Here's how the part is built. I have some questions about the finished solid (model axes, mm). A direction names the side the tool comes from. Give positions to 0.01 mm unless a question says otherwise; leave off trailing zeros. Order: outer loops, then holes, each group sorted by start corner. A loop starts at its lowest first (then second) coordinate and runs counter-clockwise, first axis right, second up. Notation, with made-up numbers: (88.25, 1) - (104.25, 1) arc R17 cw to (104.25, 15) - close; hole circle Ø3 at (88, 36.5). An arc over 180 degrees is marked (long way). One line per question, with ' | ' between items.
Autodesk Inventor part; units mm, degrees
ref_plane "YZ Plane" through (0, 0, 0) normal (1, 0, 0) x (0, 1, 0)
ref_plane "XZ Plane" through (0, 0, 0) normal (0, 1, 0) x (-1, 0, 0)
ref_plane "XY Plane" through (0, 0, 0) normal (0, 0, 1) x (1, 0, 0)
sketch "Sketch1" plane through (0, 0, 0) normal (0, 1, 0) x (-1, 0, 0)
  line L0 (52, 58.6471) -> (-48, 58.6471)
  line L1 (-48, 58.6471) -> (-48, -16.3529)
  line L2 (-48, -16.3529) -> (52, -16.3529)
  line L3 (52, -16.3529) -> (52, 58.6471)
  point P0 (0, 0)
  dimension "d0" = 100
  dimension "d1" = 75
extrude "Extrusion1" add sketch "Sketch1" along normal blind 60
sketch "Sketch2" plane through (0, 60, 0) normal (0, 1, 0) x (1, 0, 0)
  line L0 (-47, -53.6471) -> (43, -53.6471)
  line L1 (43, -53.6471) -> (43, 11.3529)
  line L2 (43, 11.3529) -> (-47, 11.3529)
  line L3 (-47, 11.3529) -> (-47, -53.6471)
  line L4 (-52, 16.3529) -> (-52, -58.6471)
  line L5 (-52, -58.6471) -> (48, -58.6471)
  line L6 (48, 16.3529) -> (-52, 16.3529)
  line L7 (48, -58.6471) -> (48, 16.3529)
  point P0 (0, 0)
  dimension "d4" = 5
  dimension "d5" = 5
  dimension "d6" = 5
  dimension "d7" = 5
extrude "Extrusion2" cut sketch "Sketch2" against normal blind 59 contours L3 L2 L1 L0
sketch "Sketch3" plane through (48, 0, -16.3529) normal (0, 0, -1) x (-1, 0, 0)
  circle A0 centre (48, 60) radius 13
  point P0 (48, 0)
  dimension "d10" = 26
  dimension "d11" = 60
sketch "Sketch13" plane through (0, 1, 0) normal (0, 1, 0) x (1, 0, 0)
  line L0 (-47, -53.6471) -> (-47, 11.3529)
  line L1 (43, 11.3529) -> (43, -53.6471)
  line L2 (-47, 11.3529) -> (43, 11.3529)
  line L3 (43, 11.3529) -> (43, -13.6471)
  line L4 (43, -13.6471) -> (-47, -13.6471)
  line L5 (-47, -13.6471) -> (-47, 11.3529)
  point P0 (0, 0)
  dimension "d44" = 25
extrude "Extrusion14" add sketch "Sketch13" along normal blind 59
sketch "Sketch14" plane through (-47, 1, 13.6471) normal (0, 0, 1) x (1, 0, 0)
  line L0 (0, 59) -> (90, 59)
  circle A0 centre (47, 59) radius 23.505
  point P0 (47, -1)
  dimension "d47" = 47.01
extrude "Extrusion15" cut sketch "Sketch14" against normal blind 12.1
sketch "Sketch15" plane through (0, 1, 0) normal (0, 1, 0) x (1, 0, 0)
  line L0 (-47, -53.6471) -> (-47, -13.6471)
  line L1 (43, -13.6471) -> (43, -53.6471)
  line L2 (-47, -53.6471) -> (43, -53.6471)
  line L3 (43, -53.6471) -> (43, -28.6471)
  line L4 (43, -28.6471) -> (-47, -28.6471)
  line L5 (-47, -28.6471) -> (-47, -53.6471)
  point P0 (0, 0)
  point P1 (-47, -28.6471)
  dimension "d50" = 25
extrude "Extrusion16" add sketch "Sketch15" along normal blind 59
sketch "Sketch16" plane through (43, 1, 28.6471) normal (0, 0, -1) x (-1, 0, 0)
  line L0 (0, 59) -> (90, 59)
  circle A0 centre (43, 59) radius 23.505
  point P0 (43, -1)
  dimension "d53" = 47.01
extrude "Extrusion17" cut sketch "Sketch16" against normal blind 12.1
sketch "Sketch17" plane through (0, 1, 0) normal (0, 1, 0) x (1, 0, 0)
  line L0 (23.505, -13.6471) -> (43, -13.6471)
  line L1 (-47, -28.6471) -> (43, -28.6471)
  line L2 (43, -28.6471) -> (43, -13.6471)
  line L3 (43, -13.6471) -> (-47, -13.6471)
  line L4 (-47, -13.6471) -> (-47, -28.6471)
  point P0 (0, 0)
extrude "Extrusion18" add sketch "Sketch17" along normal blind 59
extrude "Extrusion19" cut sketch "Sketch3" against normal blind 75
equation "\"d6\" = d5"
equation "\"d7\" = d4"
properties part number "new_box_bottom"
1) I want a section at C-C (y = 53.5). List the corners of the cut face in (x, z) for me, plus the area to 3 significant figures.
Model answer:
outline: (-52, -16.35) - (-11.26, -16.35) - (-11.26, 1.55) - (-22.59, 1.55) - (-22.59, 13.65) - (-11.26, 13.65) - (-11.26, 28.65) - (-22.59, 28.65) - (-22.59, 40.75) - (-11.26, 40.75) - (-11.26, 58.65) - (-52, 58.65) - close; (11.26, -16.35) - (48, -16.35) - (48, 58.65) - (11.26, 58.65) - (11.26, 40.75) - (22.59, 40.75) - (22.59, 28.65) - (11.26, 28.65) - (11.26, 13.65) - (22.59, 13.65) - (22.59, 1.55) - (11.26, 1.55) - close | area: 5,260 mm2
2) I want a section at B-B (z = 8.5). List the corners of the cut face in (x, y) for me (3 decimals).
Model answer:
outline: (-52, 0) - (48, 0) - (48, 60) - (23.505, 60) arc R23.505 cw to (-23.505, 60) - (-52, 60) - close
3) I want a section at D-D (z = 19). List the corners of the cut face in (x, y) for me, plus the area to 3 significant figures.
Model answer:
outline: (-52, 0) - (48, 0) - (48, 60) - (13, 60) arc R13 cw to (-13, 60) - (-52, 60) - close | area: 5,730 mm2
4) Thinking about a two-plate mould opening in Z: for faces 3 (the face through (0, 47, 21)), 4 (the face through (-0.5, 36.5, 7.7)), 5 (the face through (-1, 30, -16.353)), which applies, +Z half, -Z half, draft (parallel to the pull), parting line (faces both ways), or undercut?
Model answer:
face 3: draft | face 4: undercut | face 5: -Z half
5) Please list where these lines run through material, in increasing order: L1, parallel to Z at x = -19, y = 48.5; L2, parallel to X at y = 53.5, z = -10; L3, parallel to Y at x = 9, z = 23.
Model answer:
L1: z = -16.35 to 1.55, 13.65 to 28.65, 40.75 to 58.65 | L2: x = -52 to -11.26, 11.26 to 48 | L3: y = 0 to 50.62
6) On a 3-axis mill with a long thin cutter (end or side, diameter ignored), from which of +Z, -Z, +X, -X, +Y, -Y can I reach the whole of each face in a straight line? I mean faces 1 (the face through (-52, 30, 21)), 2 (the face through (0.5, 36.5, 34.6)). Say none if no direction works.
Model answer:
face 1: +Z, -Z, -X, +Y, -Y | face 2: +Y
7) I want a section at A-A (x = 0). List the corners of the cut face in (y, z) for me (3 decimals).
Model answer:
outline: (0, -16.353) - (47, -16.353) - (47, 1.547) - (36.495, 1.547) - (36.495, 13.647) - (47, 13.647) - (47, 28.647) - (36.495, 28.647) - (36.495, 40.747) - (47, 40.747) - (47, 58.647) - (0, 58.647) - close
